The drawing under review shows one solid part. Ordinate dimensions are in mm from its lowest x, y, z. Give positions to 0.01 mm unless a question says otherwise; leave off trailing zeros. Order: outer loops, then holes, each group sorted by start corner. A loop starts at its lowest first (then second) coordinate and runs counter-clockwise, first axis right, second up. Notation, with made-up numbers: (70, 55.5) -> (104, 55.5) arc R21 cw to (104, 89.5) -> close; hole circle Ø10 at (-18.75, 10). An arc over 180 degrees is marked (long way). Return JSON: item names as keys, results as strings. Group by question number.
1) Add section C-C (z = 2.5). State how many separate pieces and enclosed holes the cut face has, then the cut area to 3 significant figures.
2) Insertion check: P1, Ø2, axis at x = 92, z = 1.5, coming from the -Y side; P2, Ø2, axis at x = 18.5, z = 1.5, coming from the +Y side (1 decimal); P3, Ø1, axis at y = 77, z = 3, coming from the -X side. Each pin has a flat end and moves straight along its axis. Give the tip position at first contact, or say it passes through.
3) Add section D-D (x = 12.7). Give the boundary of the cut face in (y, z) (3 decimals).
4) Add section B-B (x = 93). Give the boundary of the cut face in (y, z), then the cut area to 3 significant figures.
5) To check wall thickness, follow line 1 along X through (y, z) = (12.7, 2.75) (3 decimals); line 2 along Y through (x, z) = (11, 2); line 3 along Y through (x, z) = (53, 1). State the ranges of each line that lie inside material, in increasing order.
6) Add section A-A (y = 12.7). Give the boundary of the cut face in (x, z) (3 decimals), then the cut area to 3 significant figures.
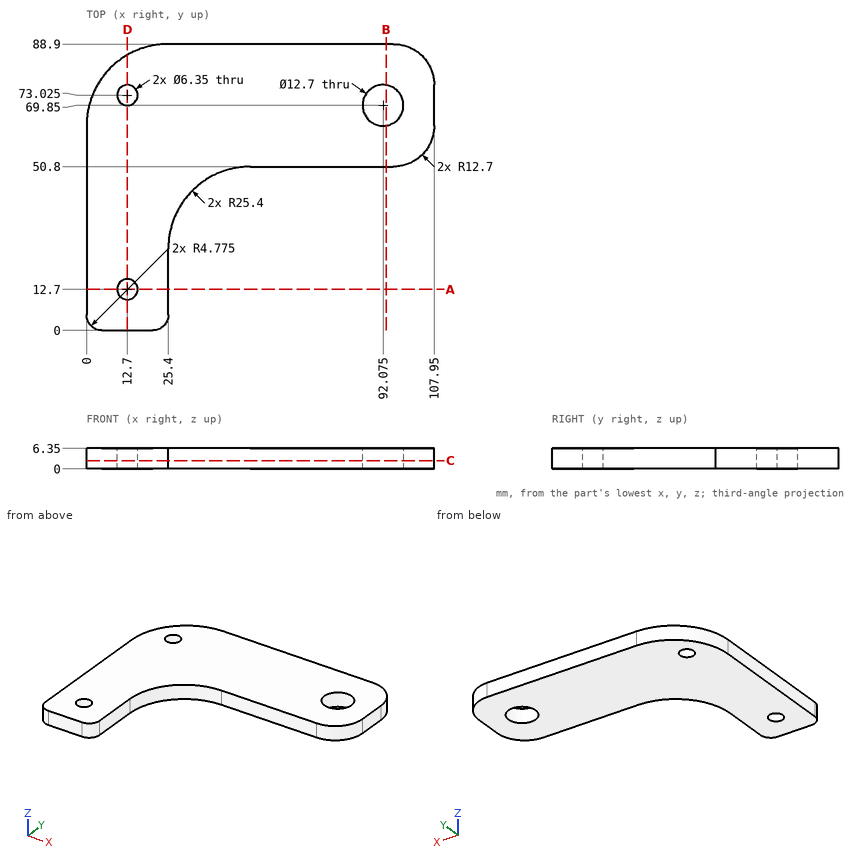
Evaluation:
{
 "1": {"separate pieces": "1", "enclosed holes": "3", "area": "5,130 mm^2"},
 "2": {"P1": "y = 50.8", "P2": "y = 88.2", "P3": "x = 3.58"},
 "3": {"outline": "(0, 0) -> (9.525, 0) -> (9.525, 6.35) -> (0, 6.35) -> close; (15.875, 0) -> (69.85, 0) -> (69.85, 6.35) -> (15.875, 6.35) -> close; (76.2, 0) -> (85.497, 0) -> (85.497, 6.35) -> (76.2, 6.35) -> close"},
 "4": {"outline": "(50.8, 0) -> (63.57, 0) -> (63.57, 6.35) -> (50.8, 6.35) -> close; (76.13, 0) -> (88.9, 0) -> (88.9, 6.35) -> (76.13, 6.35) -> close", "area": "162 mm^2"},
 "5": {"line 1": "0 to 9.525, 15.875 to 25.4", "line 2": "0 to 10.02, 15.38 to 70.34, 75.71 to 84.42", "line 3": "50.8 to 88.9"},
 "6": {"outline": "(0, 0) -> (9.525, 0) -> (9.525, 6.35) -> (0, 6.35) -> close; (15.875, 0) -> (25.4, 0) -> (25.4, 6.35) -> (15.875, 6.35) -> close", "area": "121 mm^2"}
}
